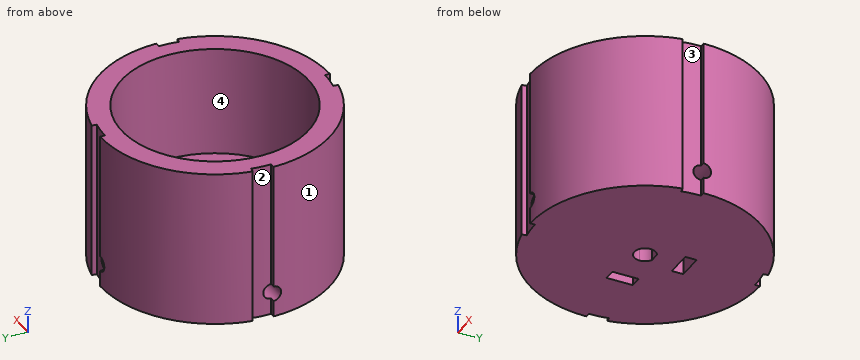
from build123d import *

# Parameters (mm, degrees)
SALIENTE_EXTRUIR1_DEPTH = 16.5
CROQUIS2_R              = 19.5
CORTAR_EXTRUIR1_DEPTH   = 23
CORTAR_EXTRUIR2_DEPTH   = 23
CROQUIS4_R              = 1.6
CORTAR_EXTRUIR3_DEPTH   = 36.5
CROQUIS5_R              = 1.6
CORTAR_EXTRUIR4_DEPTH   = 141.5
CROQUIS6_W              = 5.5
CROQUIS6_H              = 2.4
CROQUIS6_W_2            = 2.4
CROQUIS6_H_2            = 5.5
CORTAR_EXTRUIR5_DEPTH   = 283


with BuildPart() as part:
    # Croquis1 → Saliente-Extruir1 (new body, symmetric)
    with BuildSketch(Plane.XY):
        with BuildLine():
            Line((0, 24), (0, 23))
            ThreePointArc((0, 23), (2.004582083, 22.912478056), (3.993908086, 22.650578319))
            Line((3.993908086, 22.650578319), (4.167556264, 23.635386072))
            ThreePointArc((4.167556264, 23.635386072), (18.385066635, 15.426902632), (24, 0))
            Line((24, 0), (23, 0))
            ThreePointArc((23, 0), (22.912478056, -2.004582083), (22.650578319, -3.993908086))
            Line((22.650578319, -3.993908086), (23.635386072, -4.167556264))
            ThreePointArc((23.635386072, -4.167556264), (15.426902632, -18.385066635), (0, -24))
            Line((0, -24), (0, -23))
            ThreePointArc((0, -23), (-2.004582083, -22.912478056), (-3.993908086, -22.650578319))
            Line((-3.993908086, -22.650578319), (-4.167556264, -23.635386072))
            ThreePointArc((-4.167556264, -23.635386072), (-18.385066635, -15.426902632), (-24, 0))
            Line((-24, 0), (-23, 0))
            ThreePointArc((-23, 0), (-22.912478056, 2.004582083), (-22.650578319, 3.993908086))
            Line((-22.650578319, 3.993908086), (-23.635386072, 4.167556264))
            ThreePointArc((-23.635386072, 4.167556264), (-15.426902632, 18.385066635), (0, 24))
        make_face()
    extrude(amount=SALIENTE_EXTRUIR1_DEPTH, both=True)

    # Croquis2 → Cortar-Extruir1 (cut)
    with BuildSketch(Plane.XY.offset(16.5)):
        Circle(CROQUIS2_R)
    extrude(amount=-CORTAR_EXTRUIR1_DEPTH, mode=Mode.SUBTRACT)

    # Croquis3 → Cortar-Extruir2 (cut)
    with BuildSketch(Plane(origin=(0, 0, -16.5), x_dir=(-1, 0, 0), z_dir=(0, 0, -1))):
        with BuildLine():
            Line((1.030776406, 2), (-1.030776406, 2))
            ThreePointArc((-1.030776406, 2), (-1.17116461, -1.92116461), (2.25, 0))
            ThreePointArc((2.25, 0), (1.92116461, 1.17116461), (1.030776406, 2))
        make_face()
    extrude(amount=-CORTAR_EXTRUIR2_DEPTH, mode=Mode.SUBTRACT)

    # Croquis4 → Cortar-Extruir3 (cut, symmetric)
    with BuildSketch(Plane(origin=(0, 0, 0), x_dir=(1, 0, 0), z_dir=(0, 1, 0))):
        with Locations((0, 11.5)):
            Circle(CROQUIS4_R)
    extrude(amount=CORTAR_EXTRUIR3_DEPTH, both=True, mode=Mode.SUBTRACT)

    # Croquis5 → Cortar-Extruir4 (cut, symmetric)
    with BuildSketch(Plane(origin=(0, 0, 0), x_dir=(0, 0, -1), z_dir=(1, 0, 0))):
        with Locations((11.5, 0)):
            Circle(CROQUIS5_R)
    extrude(amount=CORTAR_EXTRUIR4_DEPTH, both=True, mode=Mode.SUBTRACT)

    # Croquis6 → Cortar-Extruir5 (cut)
    with BuildSketch(Plane(origin=(0, 0, -16.5), x_dir=(-1, 0, 0), z_dir=(0, 0, -1))):
        with Locations((0, 8.2)):
            Rectangle(CROQUIS6_W, CROQUIS6_H)
        with Locations((9.2, 0)):
            Rectangle(CROQUIS6_W_2, CROQUIS6_H_2)
    extrude(amount=-CORTAR_EXTRUIR5_DEPTH, mode=Mode.SUBTRACT)


solid = part.part
The model under review builds one solid part; all positions refer to its coordinate system, in mm. Face numbers are marked on the shaded views. A direction names the side the tool comes from. Round coordinates to 2 decimals unless told otherwise and drop trailing zeros. Loops run counter-clockwise (first coordinate to the right, second up) from the corner with the lowest first, then second, coordinate; pieces in that order, holes last. Notation, with made-up numbers: M 41.5,64.5 L 61.5,64.5 A12 ccw 61.5,81.5 Z; hole C 71,-6.75 d11. An arc over 180 degrees is marked long. Answer as a JSON object with one key per item and string values.
Item 1: Tool access review of the marked faces 1, 2, 3 and 4: name each direction out of +Z, -Z, +X, -X, +Y, -Y from which nothing blocks a thin tool from reaching the whole face with its end or side.
Check sheet entries:
{"face 1": "+Z, -Z, -X, -Y", "face 2": "+Z, -Z, -X", "face 3": "+Z, -Z, +X", "face 4": "+Z"}
Item 2: We need section A-A, the plane z = -2. State the section outline as (x, y) points.
Check sheet entries:
{"outline": "M -24,0 A24 ccw -4.17,-23.64 L -3.99,-22.65 A23 ccw 0,-23 L 0,-24 A24 ccw 23.64,-4.17 L 22.65,-3.99 A23 ccw 23,0 L 24,0 A24 ccw 4.17,23.64 L 3.99,22.65 A23 ccw 0,23 L 0,24 A24 ccw -23.64,4.17 L -22.65,3.99 A23 ccw -23,0 Z; hole C 0,0 d39"}
Item 3: We need section B-B, the plane x = -14. State the section outline as (y, z) points, and give its area (3 significant figures).
Check sheet entries:
{"outline": "M -19.49,-16.5 L 19.49,-16.5 L 19.49,16.5 L 13.57,16.5 L 13.57,-6.5 L -13.57,-6.5 L -13.57,16.5 L -19.49,16.5 Z; hole C 0,-11.5 d3.2", "area": "654 mm2"}
Item 4: For line 1 along Z through (x, y) = (0, 13.75); line 2 along Z through (x, y) = (-5.5, 16); line 3 along Y through (x, z) = (-14, -2), list the stretches that pass through material, from the lowest coordinate up.
Check sheet entries:
{"line 1": "-16.5 to -13.1, -9.9 to -6.5", "line 2": "-16.5 to -6.5", "line 3": "-19.49 to -13.57, 13.57 to 19.49"}
Item 5: Clearance check with flat-ended pins moving along their axes: P1, Ø2, axis at x = 1, y = 18, coming from the +Z side; P2, Ø5, axis at y = 15, z = -4, coming from the -X side; P3, Ø1.5, axis at x = -15.5, z = 11, coming from the +Y side. State where each tip first meets the part, or that it passes through.
Check sheet entries:
{"P1": "z = -6.5", "P2": "x = -20.49", "P3": "y = 18.93"}
